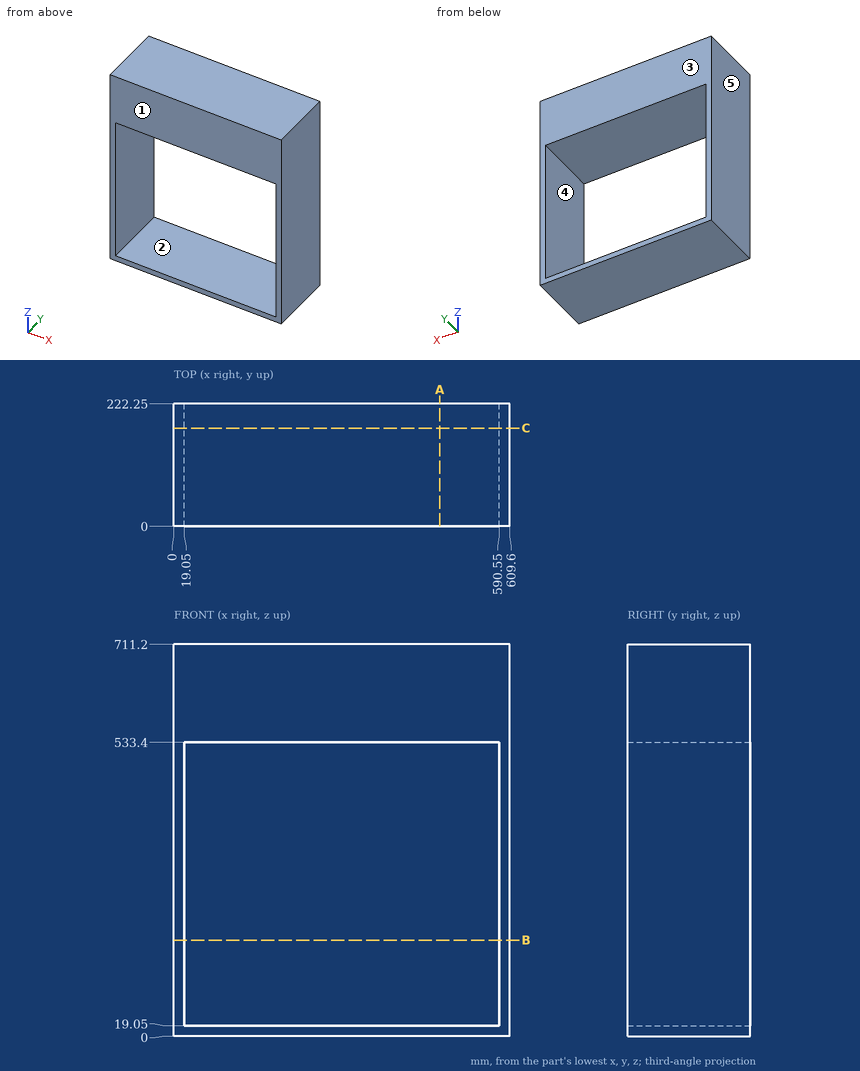
The drawing under review shows one solid part. Ordinate dimensions are in mm from its lowest x, y, z. A direction names the side the tool comes from. Coordinates: 2 decimals unless noted, no trailing zeros. Write each loop counter-clockwise with the first axis right and the second up, starting at its lowest first coordinate (ties: lowest second). Pieces come first, ordered by that corner, then holes.
1) Add section B-B (z = 174). Write out the cut boundary in (x, y), plus the area to 3 significant figures.
2) Machinability: for the marked faces 1 and 2, which of the approach directions +Z, -Z, +X, -X, +Y, -Y give a long, thin tool a straight path to every point of the face, cutting with its end or side? Answer none if there is none.
3) Add section C-C (y = 178.5). Write out the cut boundary in (x, z).
4) Mouldability with a two-part tool opening along X and no side actions: class the marked faces 3, 4 and 5 as +X half, -X half, draft (parallel to the pull), parting line (faces both ways), or undercut.
5) To check wall thickness, follow L1, parallel to Z at x = 119, y = 78.5; L2, parallel to X at y = 130, z = 62. State the ranges of each line that lie inside material, in increasing order.
6) Add section A-A (x = 483). Write out the cut boundary in (y, z).
Check result:
1. outline: (0, 0) - (19.05, 0) - (19.05, 222.25) - (0, 222.25) - close; (590.55, 0) - (609.6, 0) - (609.6, 222.25) - (590.55, 222.25) - close
1. area: 8,470 mm2
2. face 1: +Z, -Z, +X, -X, -Y
2. face 2: +Y, -Y
3. outline: (0, 0) - (609.6, 0) - (609.6, 711.2) - (0, 711.2) - close; hole (19.05, 19.05) - (590.55, 19.05) - (590.55, 533.4) - (19.05, 533.4) - close
4. face 3: draft
4. face 4: undercut
4. face 5: -X half
5. L1: z = 0 to 19.05, 533.4 to 711.2
5. L2: x = 0 to 19.05, 590.55 to 609.6
6. outline: (0, 0) - (222.25, 0) - (222.25, 19.05) - (0, 19.05) - close; (0, 533.4) - (222.25, 533.4) - (222.25, 711.2) - (0, 711.2) - close
